```python
from build123d import *

# Parameters (mm, degrees)
EXTRUDE_2_DEPTH     = 7
SKETCH_2_10_R       = 5
EXTRUDE_6_DEPTH     = 3
EXTRUDE_7_DEPTH     = 1
SKETCH_5_R          = 3
CUT_EXTRUDE_1_DEPTH = 3
SKETCH_5_5_R        = 3
CUT_EXTRUDE_2_DEPTH = 6
FILLET_1_R          = 3
CHAMFER_2_SIZE      = 0.5


with BuildPart() as part:
    # Sketch 2 → Extrude 2 (new body, symmetric)
    with BuildSketch(Plane.XY):
        Polygon((5, 21.609375634), (5, 10.923979425), (5, 0), (0, 0), (0, 88), (5, 88), (5, 78), (5, 68), align=None)
    extrude(amount=EXTRUDE_2_DEPTH, both=True)

    # Sketch 2_10 → Extrude 6 (add, symmetric)
    with BuildSketch(Plane.XY):
        with BuildLine():
            Line((8, 75), (80, 75))
            ThreePointArc((80, 75), (87.071067812, 72.071067812), (90, 65))
            Line((90, 65), (90, 62.305456282))
            ThreePointArc((90, 62.305456282), (85.557698692, 48.079387798), (73.80951804, 38.909037925))
            Line((73.80951804, 38.909037925), (6.942857835, 13.731549628))
            ThreePointArc((6.942857835, 13.731549628), (5.533076157, 12.631107643), (5, 10.923979425))
            Line((5, 10.923979425), (5, 21.609375634))
            ThreePointArc((5, 21.609375634), (6.292871782, 19.142451791), (9.057142165, 18.801805431))
            Line((9.057142165, 18.801805431), (63.057142165, 39.134574615))
            ThreePointArc((63.057142165, 39.134574615), (64.466923843, 40.2350166), (65, 41.942144818))
            Line((65, 41.942144818), (65, 55))
            ThreePointArc((65, 55), (67.928932188, 62.071067812), (75, 65))
            Line((75, 65), (82, 65))
            ThreePointArc((82, 65), (85, 68), (82, 71))
            Line((82, 71), (8, 71))
            ThreePointArc((8, 71), (5.878679656, 70.121320344), (5, 68))
            Line((5, 68), (5, 78))
            ThreePointArc((5, 78), (5.878679656, 75.878679656), (8, 75))
        make_face()
        with Locations((75, 55)):
            Circle(SKETCH_2_10_R, mode=Mode.SUBTRACT)
    extrude(amount=EXTRUDE_6_DEPTH, both=True)

    # Sketch 2_11 → Extrude 7 (add, symmetric)
    with BuildSketch(Plane.XY):
        with BuildLine():
            ThreePointArc((5, 68), (5.878679656, 70.121320344), (8, 71))
            Line((8, 71), (82, 71))
            ThreePointArc((82, 71), (85, 68), (82, 65))
            Line((82, 65), (75, 65))
            ThreePointArc((75, 65), (67.928932188, 62.071067812), (65, 55))
            Line((65, 55), (65, 41.942144818))
            ThreePointArc((65, 41.942144818), (64.466923843, 40.2350166), (63.057142165, 39.134574615))
            Line((63.057142165, 39.134574615), (9.057142165, 18.801805431))
            ThreePointArc((9.057142165, 18.801805431), (6.292871782, 19.142451791), (5, 21.609375634))
            Line((5, 21.609375634), (5, 68))
        make_face()
    extrude(amount=EXTRUDE_7_DEPTH, both=True)

    # Sketch 5 → Cut-Extrude 1 (cut)
    with BuildSketch(Plane(origin=(5, 0, 0), x_dir=(0, 0, -1), z_dir=(1, 0, 0))):
        with BuildLine():
            Line((-5, 88), (-5, 83))
            ThreePointArc((-5, 83), (0, 78), (5, 83))
            Line((5, 83), (5, 88))
            Line((5, 88), (-5, 88))
        make_face()
        with Locations((0, 83)):
            Circle(SKETCH_5_R, mode=Mode.SUBTRACT)
        with BuildLine():
            Line((-5, 5), (-5, 0))
            Line((-5, 0), (5, 0))
            Line((5, 0), (5, 5))
            ThreePointArc((5, 5), (0, 10), (-5, 5))
        make_face()
        with Locations((0, 5)):
            Circle(SKETCH_5_R, mode=Mode.SUBTRACT)
    extrude(amount=-CUT_EXTRUDE_1_DEPTH, mode=Mode.SUBTRACT)

    # Sketch 5_5 → Cut-Extrude 2 (cut, through all)
    with BuildSketch(Plane(origin=(5, 0, 0), x_dir=(0, 0, -1), z_dir=(1, 0, 0))):
        with Locations((0, 83)):
            Circle(SKETCH_5_5_R)
        with Locations((0, 5)):
            Circle(SKETCH_5_5_R)
    extrude(amount=-CUT_EXTRUDE_2_DEPTH, mode=Mode.SUBTRACT)

    # Fillet 1
    fillet_1_edges = [part.edges().sort_by_distance(p)[0] for p in [
        (2.5, 0, 7),
        (2.5, 0, -7),
        (2.5, 88, -7),
        (2.5, 88, 7),
    ]]
    fillet(fillet_1_edges, radius=FILLET_1_R)

    # Chamfer 2
    chamfer_2_edges = [part.edges().sort_by_distance(p)[0] for p in [
        (70, 55, 3),
        (70, 55, -3),
    ]]
    chamfer(chamfer_2_edges, length=CHAMFER_2_SIZE)


solid = part.part
```
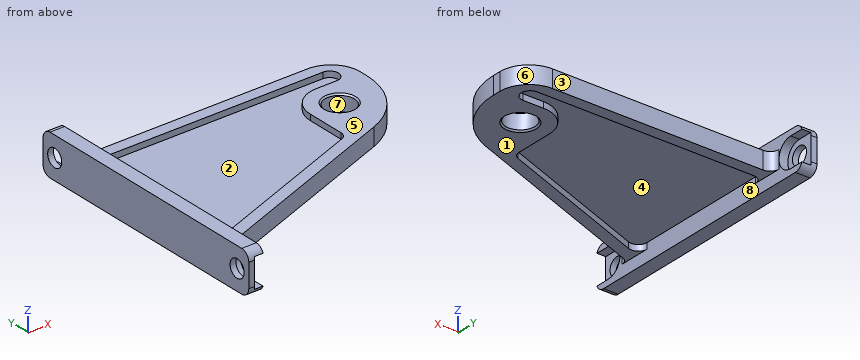
The model under review builds one solid part; all positions refer to its coordinate system, in mm. Face numbers are marked on the shaded views. A direction names the side the tool comes from. Give positions to 0.01 mm unless a question says otherwise; leave off trailing zeros. Write each loop counter-clockwise with the first axis right and the second up, starting at its lowest first coordinate (ties: lowest second). Pieces come first, ordered by that corner, then holes. Notation, with made-up numbers: (47, 89) -> (67, 89) arc R12 cw to (67, 94) -> close; hole circle Ø8 at (39.25, 40). An arc over 180 degrees is marked (long way). Put each result on its own line as item: value.
(1) We need section B-B, the plane y = 36. Give the boundary of the cut face in (x, z), and give its area (3 significant figures).
Results are:
outline: (0, -7) -> (5, -7) -> (5, -1) -> (54.73, -1) -> (54.73, -3) -> (66.08, -3) -> (66.08, 3) -> (54.73, 3) -> (54.73, 1) -> (5, 1) -> (5, 7) -> (0, 7) -> close
area: 238 mm²
(2) To check wall thickness, follow probe 1 along Y at (x, z) = (1.1, 0); probe 2 along Y at (x, z) = (79.5, 2); probe 3 along Z at (x, y) = (63.5, 72.5). State the ranges of each line that lie inside material, in increasing order. Write a range as from..to.
Results are:
probe 1: 0..2, 8..80, 86..88
probe 2: 41.94..52.82, 57.18..65, 71..75
probe 3: -3..3
(3) Tool access review of the marked faces 1, 2, 3 and 4: name each direction out of +Z, -Z, +X, -X, +Y, -Y from which nothing blocks a thin tool from reaching the whole face with its end or side.
Results are:
face 1: -Z, +X, +Y, -Y
face 2: +Z
face 3: +Z, -Z, +X, +Y
face 4: -Z
(4) For pin 1 Ø8 at (y, z) = (81.5, 1) entering from +X; pin 2 Ø11.5 at (x, y) = (75, 55) entering from +Z; pin 3 Ø4 at (x, z) = (50.5, -2) entering from -Y, all flat-tipped, find the tip position at first contact; note any pin that passes through.
Results are:
pin 1: x = 5.04
pin 2: z = 3
pin 3: y = 29.38
(5) We need section A-A, the plane x = 15.5. Give the boundary of the cut face in (y, z).
Results are:
outline: (16.95, -3) -> (21.23, -3) -> (21.23, -1) -> (71, -1) -> (71, -3) -> (75, -3) -> (75, 3) -> (71, 3) -> (71, 1) -> (21.23, 1) -> (21.23, 3) -> (16.95, 3) -> close
(6) The part is to be moulded in two halves that separate along Y. For the marked faces 5, 6, 7 and 8, say which applies: pulls with the +Y half, pulls with the -Y half, needs draft (parallel to the pull), parting line crosses it, or undercut.
Results are:
face 5: needs draft
face 6: pulls with the +Y half
face 7: undercut
face 8: undercut
